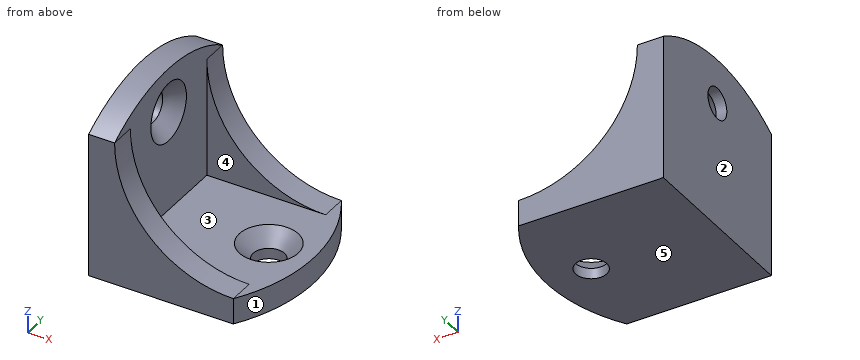
```python
from build123d import *

# Parameters (mm, degrees)
BOSS_EXTRUDE1_DEPTH          = 12
BOSS_EXTRUDE1_DEPTH_BACK     = 12
BOSS_EXTRUDE2_DEPTH          = 3.5
CUT_EXTRUDE3_START           = -4.5
CUT_EXTRUDE3_DEPTH           = 25
CUT_EXTRUDE1_START           = -4.5
SKETCH5_R                    = 2.1
CUT_EXTRUDE1_DEPTH           = 25
SKETCH6_R                    = 3.9624
CUT_EXTRUDE2_DEPTH           = 3.5
CUT_EXTRUDE2_TAPER           = 42
CUT_EXTRUDE2_OTHER_WAY_DEPTH = 3.048
CUT_EXTRUDE2_OTHER_WAY_TAPER = 42
CIRPATTERN2_COUNT            = 2
CIRPATTERN2_ANGLE            = 180


with BuildPart() as part:
    # Sketch3 → Boss-Extrude1 (new body, two sides)
    with BuildSketch(Plane(origin=(0, 0, 0), x_dir=(1, 0, 0), z_dir=(0, 1, 0))) as boss_extrude1_sk:
        Polygon((0, -23), (3.5, -23), (3.5, -3.5), (23, -3.5), (23, 0), (0, 0), align=None)
    extrude(amount=BOSS_EXTRUDE1_DEPTH)
    extrude(boss_extrude1_sk.sketch, amount=-BOSS_EXTRUDE1_DEPTH_BACK)

    # Sketch8 → Boss-Extrude2 (add)
    with BuildSketch(Plane(origin=(0, 12, 0), x_dir=(1, 0, 0), z_dir=(0, 1, 0))):
        with BuildLine():
            Line((3.5, -3.5), (19.5, -3.5))
            ThreePointArc((19.5, -3.5), (8.186291501, -8.186291501), (3.5, -19.5))
            Line((3.5, -19.5), (3.5, -3.5))
        make_face()
    boss_extrude2 = extrude(amount=-BOSS_EXTRUDE2_DEPTH)

    # Mirror1: Boss-Extrude2 across plane
    add(boss_extrude2.mirror(Plane.ZX))

    # Sketch7 → Cut-Extrude3 (cut)
    with BuildSketch(Plane(origin=(3.5, 0, 0), x_dir=(0, 0, -1), z_dir=(1, 0, 0)).offset(CUT_EXTRUDE3_START)):
        with BuildLine():
            Line((19.124723765, 72.581039953), (-19.5, 12))
            ThreePointArc((-19.5, 12), (-23, 0), (-19.5, -12))
            Line((-19.5, -12), (19.124723765, -72.581039953))
            Line((19.124723765, -72.581039953), (-124.568445004, -72.581039953))
            Line((-124.568445004, -72.581039953), (-124.568445004, 72.581039953))
            Line((-124.568445004, 72.581039953), (19.124723765, 72.581039953))
        make_face()
    cut_extrude3 = extrude(amount=CUT_EXTRUDE3_DEPTH, mode=Mode.SUBTRACT)

    # Sketch5 → Cut-Extrude1 (cut)
    with BuildSketch(Plane(origin=(3.5, 0, 0), x_dir=(0, 0, -1), z_dir=(1, 0, 0)).offset(CUT_EXTRUDE1_START)):
        with Locations((-17, 0)):
            Circle(SKETCH5_R)
    cut_extrude1 = extrude(amount=CUT_EXTRUDE1_DEPTH, mode=Mode.SUBTRACT)

    # Sketch6 → Cut-Extrude2 (cut)
    with BuildSketch(Plane(origin=(3.5, 0, 0), x_dir=(0, 0, -1), z_dir=(1, 0, 0))):
        with Locations((-17, 0)):
            Circle(SKETCH6_R)
    cut_extrude2 = extrude(amount=-CUT_EXTRUDE2_DEPTH, taper=CUT_EXTRUDE2_TAPER, mode=Mode.SUBTRACT)

    # Sketch6 → Cut-Extrude2 other way (cut)
    with BuildSketch(Plane(origin=(3.5, 0, 0), x_dir=(0, 0, -1), z_dir=(1, 0, 0))):
        with Locations((-17, 0)):
            Circle(SKETCH6_R)
    extrude(amount=CUT_EXTRUDE2_OTHER_WAY_DEPTH, taper=CUT_EXTRUDE2_OTHER_WAY_TAPER, mode=Mode.SUBTRACT)

    # CirPattern2: Cut-Extrude3, Cut-Extrude1, Cut-Extrude2 ×2 about axis
    cirpattern2_axis = Axis((0, 0, 0), (0.707106781, 0, 0.707106781))
    for i in range(1, CIRPATTERN2_COUNT):
        add(cut_extrude3.rotate(cirpattern2_axis, i * CIRPATTERN2_ANGLE / (CIRPATTERN2_COUNT - 1)), mode=Mode.SUBTRACT)
        add(cut_extrude1.rotate(cirpattern2_axis, i * CIRPATTERN2_ANGLE / (CIRPATTERN2_COUNT - 1)), mode=Mode.SUBTRACT)
        add(cut_extrude2.rotate(cirpattern2_axis, i * CIRPATTERN2_ANGLE / (CIRPATTERN2_COUNT - 1)), mode=Mode.SUBTRACT)


solid = part.part
```
The model under review builds one solid part; all positions refer to its coordinate system, in mm. Face numbers are marked on the shaded views. A direction names the side the tool comes from. Give positions to 0.01 mm unless a question says otherwise; leave off trailing zeros. Write each loop counter-clockwise with the first axis right and the second up, starting at its lowest first coordinate (ties: lowest second). Pieces come first, ordered by that corner, then holes.
(1) Tool access review of the marked faces 4 and 5: name each direction out of +Z, -Z, +X, -X, +Y, -Y from which nothing blocks a thin tool from reaching the whole face with its end or side.
(2) The part is to be moulded in two halves that separate along Y. For the marked faces 1, 2 and 3, say which applies: released by +Y, released by -Y, zero draft, split by the parting line, or undercut.
(3) Consider section B-B, the plane y = 0. Give the number of separate pieces and of enclosed holes in the cut face, and give its area (3 significant figures).
(4) Consider section C-C, the plane x = 17. Give the boundary of the cut face in (y, z), and give its area (3 significant figures).
(5) Consider section A-A, the plane z = 17. Give the boundary of the cut face in (x, y).
(6) For P1, Ø1.5, axis at y = 6.5, z = 19, coming from the +X side; P2, Ø2.5, axis at x = 17, y = 0, coming from the +Z side; P3, Ø10, axis at x = 14.5, y = 9, coming from the +Z side; P4, Ø5, axis at x = 10, y = 3, coming from the +Z side, all flat-tipped, find the tip position at first contact; note any pin that passes through.
(7) Consider section D-D, the plane x = 7.75. Give the boundary of the cut face in (y, z).
(8) To check wall thickness, follow L1, parallel to Y at x = 17, z = 0.9; L2, parallel to Y at x = 4.75, z = 6.5; L3, parallel to X at y = -7.5, z = 9. State the ranges of each line that lie inside material, in increasing order.
Returned:
1. face 4: +Z, +X
1. face 5: -Z, +X, -X, +Y, -Y
2. face 1: split by the parting line
2. face 2: zero draft
2. face 3: undercut
3. separate pieces: 3
3. enclosed holes: 0
3. area: 112 mm2
4. outline: (-12, 0) - (-2.1, 0) - (-2.1, 1.43) - (-3.96, 3.5) - (-8.5, 3.5) - (-8.5, 3.7) - (-12, 3.7) - close; (2.1, 0) - (12, 0) - (12, 3.7) - (8.5, 3.7) - (8.5, 3.5) - (3.96, 3.5) - (2.1, 1.43) - close
4. area: 66.8 mm2
5. outline: (0, -12) - (3.7, -12) - (3.7, -8.5) - (3.5, -8.5) - (3.5, -3.96) - (1.43, -2.1) - (0, -2.1) - close; (0, 2.1) - (1.43, 2.1) - (3.5, 3.96) - (3.5, 8.5) - (3.7, 8.5) - (3.7, 12) - (0, 12) - close
6. P1: stops at x = 3.5
6. P2: passes through
6. P3: stops at z = 7.01
6. P4: stops at z = 3.5
7. outline: (-12, 0) - (12, 0) - (12, 8.64) - (8.5, 8.64) - (8.5, 3.5) - (-8.5, 3.5) - (-8.5, 8.64) - (-12, 8.64) - close
8. L1: y = -12 to -2.1, 2.1 to 12
8. L2: y = -12 to -8.5, 8.5 to 12
8. L3: x = 0 to 3.5
